```python
from build123d import *

# Parameters (mm, degrees)
SKETCH006_R      = 3
EXTRUDE004_DEPTH = 6
SKETCH004_R      = 3
EXTRUDE003_DEPTH = 6
SKETCH005_R      = 3
EXTRUDE005_DEPTH = 6


with BuildPart() as der:
    # Sketch006 → Extrude004 (new body)
    with BuildSketch(Plane(origin=(0, 0, 0), x_dir=(0, -1, 0), z_dir=(-1, 0, 0))):
        with BuildLine():
            ThreePointArc((-10.803604, 3.701349), (-16.887759, 1.835055), (-15.021464, -4.2491))
            Line((-15.021464, -4.2491), (37.981534, -32.368171))
            ThreePointArc((37.981534, -32.368171), (44.065689, -30.501877), (42.199395, -24.417722))
            Line((-10.803604, 3.701349), (42.199395, -24.417722))
        make_face()
        with Locations((-12.912534, -0.273875)):
            Circle(SKETCH006_R, mode=Mode.SUBTRACT)
        with Locations((40.090464, -28.392947)):
            Circle(SKETCH006_R, mode=Mode.SUBTRACT)
    extrude(amount=EXTRUDE004_DEPTH)


with BuildPart() as arriba:
    # Sketch004 → Extrude003 (new body)
    with BuildSketch(Plane(origin=(0, 0, 0), x_dir=(0, -1, 0), z_dir=(-1, 0, 0))):
        with BuildLine():
            ThreePointArc((-12.757495, 4.884875), (-17.769398, -0.109168), (-12.769395, -5.115125))
            Line((-12.769395, -5.115125), (52.23079, -5.115125))
            ThreePointArc((52.23079, -5.115125), (57.153448, -0.19832), (52.242505, 4.730186))
            Line((-12.757495, 4.884875), (52.242505, 4.730186))
        make_face()
        with Locations((-12.769395, -0.115118)):
            Circle(SKETCH004_R, mode=Mode.SUBTRACT)
        with Locations((52.23079, -0.192462)):
            Circle(SKETCH004_R, mode=Mode.SUBTRACT)
    extrude(amount=EXTRUDE003_DEPTH)


with BuildPart() as obj1:
    # Sketch005 → Extrude005 (new body)
    with BuildSketch(Plane(origin=(0, 0, 0), x_dir=(0, -1, 0), z_dir=(-1, 0, 0))):
        with BuildLine():
            ThreePointArc((56.876804, -2.145211), (54.255545, 4.422056), (47.688278, 1.800797))
            Line((47.688278, 1.800797), (35.731876, -26.04044))
            ThreePointArc((35.731876, -26.04044), (38.353136, -32.607707), (44.920403, -29.986447))
            Line((56.876804, -2.145211), (44.920403, -29.986447))
        make_face()
        with Locations((40.326139, -28.013444)):
            Circle(SKETCH005_R, mode=Mode.SUBTRACT)
        with Locations((52.282541, -0.172207)):
            Circle(SKETCH005_R, mode=Mode.SUBTRACT)
    extrude(amount=EXTRUDE005_DEPTH)

    # Fusion018: union Der, arriba
    add(der.part)
    add(arriba.part)


with BuildPart() as obj1_1:
    # Fusion018 placement: moved
    add(obj1.part.moved(Location((54, 57.6, 173.85))))


solid = obj1_1.part
```
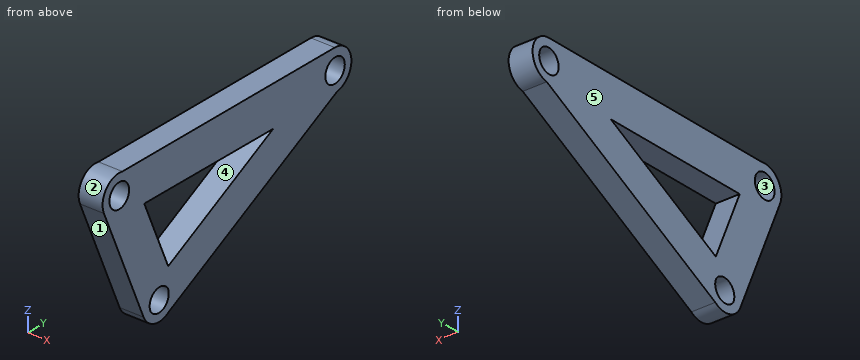
Source: CAD feature listing. Evaluate the final solid. Frame: model axes, mm. Face numbers are marked on the shaded views. A direction names the side the tool comes from. Give positions to 0.01 mm unless a question says otherwise; leave off trailing zeros. Loops run counter-clockwise (first coordinate to the right, second up) from the corner with the lowest first, then second, coordinate; pieces in that order, holes last. Notation, with made-up numbers: M 73.5,-2.75 L 78.5,-2.75 A19 ccw 78.5,21.25 Z; hole C -32,-16.75 d6. An arc over 180 degrees is marked long. Put each result on its own line as item: value.
Q1. Section A-A (y = 35). Return the cut outline in (x, z), and give its area (3 significant figures).
Response values:
outline: M 48,149.64 L 54,149.64 L 54,159.83 L 48,159.83 Z; M 48,168.73 L 54,168.73 L 54,178.65 L 48,178.65 Z
area: 121 mm²
Q2. Mould query, pull axis Z, two halves, no side actions, for the marked faces 1, 2 and 3. Classes: released by +Z, released by -Z, zero draft, split by the parting line, or undercut.
Response values:
face 1: released by -Z
face 2: split by the parting line
face 3: undercut
Q3. Section B-B (x = 50.4). Return the cut outline in (y, z) (1 decimal).
Response values:
outline: M 0.7,171.7 L 12.7,143.9 A5 ccw 20.2,141.8 L 71.1,168.8 A5 ccw 70.4,178.7 L 6.3,178.6 A5 ccw Z; hole M 4.2,170.9 A3 ccw 6.4,176.5 A3 ccw Z; hole M 12.9,168.7 L 20.1,151.9 L 51.8,168.7 Z; hole M 14.9,144.1 A3 ccw 19.9,147.2 A3 ccw Z; hole M 68.2,171.6 A3 ccw 72.7,175.7 A3 ccw Z
Q4. Section C-C (z = 164.5). Return the cut outline in (x, y), and give its area (3 significant figures).
Response values:
outline: M 48,3.82 L 54,3.82 L 54,14.7 L 48,14.7 Z; M 48,43.8 L 54,43.8 L 54,63.01 L 48,63.01 Z
area: 181 mm²
Q5. Line query: probe 1 along Z at (x, y) = (51.4, 71.5); probe 2 along Z at (x, y) = (52.9, 26.5); probe 3 along Y at (x, z) = (49.65, 175). Output: solid intervals per line, ascending. Write a range as [from, to].
Response values:
probe 1: z = [168.86, 170.96], [176.41, 178.61]
probe 2: z = [145.13, 155.32], [168.73, 178.63]
probe 3: y = [0.5, 2.69], [8.01, 67.87], [73.09, 75.21]
Q6. Pin query (flat end, axial travel): P1, Ø1, axis at x = 51.5, z = 154.5, coming from the +Y side; P2, Ø1.5, axis at x = 50.5, y = 29.5, coming from the -Z side; P3, Ø12, axis at y = 43, z = 165, coming from the +X side; P4, Ø3, axis at x = 50, z = 151, coming from the +Y side. Return the tip coordinate at first contact, or that it passes through.
Response values:
P1: stops at y = 45.1
P2: stops at z = 146.33
P3: stops at x = 54
P4: stops at y = 40.39
Q7. Section D-D (y = 11). Return the cut outline in (x, z).
Response values:
outline: M 48,147.77 L 54,147.77 L 54,178.59 L 48,178.59 Z
Q8. Reachability of the marked faces 4 and 5 from +Z, -Z, +X, -X, +Y, -Y: full face, straight path, thin tool, end or side. Return the list, or none.
Response values:
face 4: +X, -X
face 5: +Z, -Z, -X, +Y, -Y
